Check sheet for the modelled part. Datum: model origin and axes. Units: mm. Face numbers are marked on the shaded views. Round coordinates to 2 decimals unless told otherwise and drop trailing zeros. Order: outer loops, then holes, each group sorted by start corner. A loop starts at its lowest first (then second) coordinate and runs counter-clockwise, first axis right, second up. Notation, with made-up numbers: (-29.5, -32) -> (28.5, -32) arc R17 ccw to (28.5, -11) -> close; hole circle Ø7 at (-10, 7.5). An arc over 180 degrees is marked (long way). Answer in a Markdown table with one row per item.
from build123d import *

# Parameters (mm, degrees)
PAD_DEPTH           = 3
PAD001_DEPTH        = 3.6
PAD002_DEPTH        = 5
HOLE001_D           = 3.3
HOLE001_DEPTH       = 25
HOLE001_CSINK_D     = 6
HOLE001_CSINK_ANGLE = 90
HOLE_D              = 3.3
HOLE_DEPTH          = 25
HOLE_CSINK_D        = 6
HOLE_CSINK_ANGLE    = 90


with BuildPart() as part:
    # Sketch → Pad (new body)
    with BuildSketch(Plane.XY):
        with BuildLine():
            Line((-31.5, 8.75), (-10.25, 8.75))
            ThreePointArc((-10.25, 8.75), (0, -1.5), (10.25, 8.75))
            Line((10.25, 8.75), (31.5, 8.75))
            Line((31.5, 8.75), (31.5, -8.75))
            Line((31.5, -8.75), (-31.5, -8.75))
            Line((-31.5, -8.75), (-31.5, 8.75))
        make_face()
    extrude(amount=PAD_DEPTH)

    # Sketch001 (on Face8 of Pad) → Pad001 (join)
    with BuildSketch(Plane.XY.offset(3)):
        Polygon((8.25, -5.539419), (16.5, 8.75), (31.5, 8.75), (31.5, -8.75), (-31.5, -8.75), (-31.5, 8.75), (-16.5, 8.75), (-8.25, -5.539419), align=None)
    extrude(amount=PAD001_DEPTH)

    # Sketch002 (on Face15 of Pad001) → Pad002 (join)
    with BuildSketch(Plane.XY.offset(6.6)):
        with BuildLine():
            Line((-31.5, 8.75), (-13.25, 8.75))
            ThreePointArc((-13.25, 8.75), (0, -4.5), (13.25, 8.75))
            Line((13.25, 8.75), (31.5, 8.75))
            Line((31.5, 8.75), (31.5, -8.75))
            Line((31.5, -8.75), (-31.5, -8.75))
            Line((-31.5, -8.75), (-31.5, 8.75))
        make_face()
    extrude(amount=PAD002_DEPTH)

    # Hole001
    with Locations(Plane.XY.offset(11.6)):
        with Locations((-22.54, -1.95), (22.54, -1.95)):
            CounterSinkHole(HOLE001_D / 2, HOLE001_CSINK_D / 2, depth=HOLE001_DEPTH, counter_sink_angle=HOLE001_CSINK_ANGLE)

    # Hole
    with Locations(Plane.XZ.offset(8.75)):
        with Locations((26.5, 4.5), (-26.5, 4.5)):
            CounterSinkHole(HOLE_D / 2, HOLE_CSINK_D / 2, depth=HOLE_DEPTH, counter_sink_angle=HOLE_CSINK_ANGLE)


solid = part.part
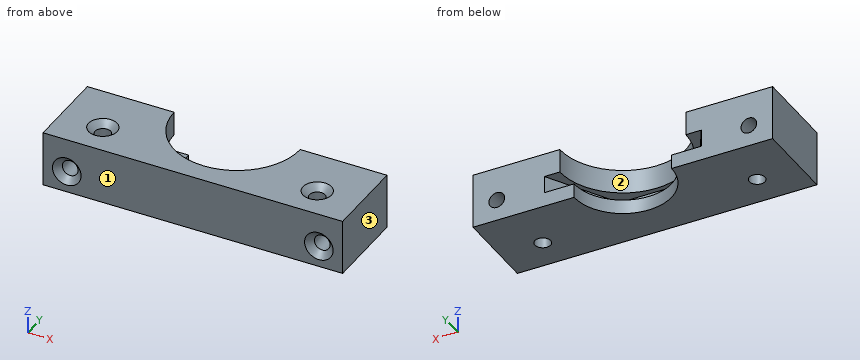
Item 1: Mould release check, pull along X, two halves, no side actions. Record for the marked faces 1, 2 and 3: pulls with the +X half, pulls with the -X half, needs draft (parallel to the pull), parting line crosses it, or undercut.
Result sheet:
| item | result |
|---|---|
| face 1 | needs draft |
| face 2 | undercut |
| face 3 | pulls with the +X half |
Item 2: Depth check by flat-ended pin: P1, Ø1.1, axis at x = 1.5, z = 5, coming from the +Y side; P2, Ø4, axis at x = 26.5, z = 4.5, coming from the -Y side; P3, Ø4, axis at x = 22.54, y = -1.95, coming from the +Z side; P4, Ø2, axis at x = -22.54, y = -1.95, coming from the +Z side. Enter the tip coordinate at first touch or a pass-through.
Result sheet:
| item | result |
|---|---|
| P1 | stops at y = -5.54 |
| P2 | stops at y = -7.75 |
| P3 | stops at z = 10.6 |
| P4 | passes through |
Item 3: Cross-section at B-B (x = -22.54). Record the boundary of the cut face in (y, z), and give its area (3 significant figures).
Result sheet:
| item | result |
|---|---|
| outline | (-8.75, 0) -> (-3.6, 0) -> (-3.6, 10.25) -> (-4.95, 11.6) -> (-8.75, 11.6) -> close; (-0.3, 0) -> (8.75, 0) -> (8.75, 11.6) -> (1.05, 11.6) -> (-0.3, 10.25) -> close |
| area | 163 mm^2 |
Item 4: Cross-section at D-D (y = 4.75). Record the boundary of the cut face in (x, z), and give its area (3 significant figures).
Result sheet:
| item | result |
|---|---|
| outline | (-31.5, 0) -> (-9.44, 0) -> (-9.44, 3) -> (-14.19, 3) -> (-14.19, 6.6) -> (-12.63, 6.6) -> (-12.63, 11.6) -> (-31.5, 11.6) -> close; (9.44, 0) -> (31.5, 0) -> (31.5, 11.6) -> (12.63, 11.6) -> (12.63, 6.6) -> (14.19, 6.6) -> (14.19, 3) -> (9.44, 3) -> close; hole circle Ø3.3 at (-26.5, 4.5); hole circle Ø3.3 at (26.5, 4.5) |
| area | 429 mm^2 |
Item 5: Scan lines: line 1 (X direction, y = -1.95, z = 2.5); line 2 (Y direction, x = -22.54, z = 7.75); line 3 (X direction, y = -1.5, z = 8.5). Record each from-to range of solid material in increasing order. Write a range as [from, to].
Result sheet:
| item | result |
|---|---|
| line 1 | x = [-31.5, -24.19], [-20.89, 20.89], [24.19, 31.5] |
| line 2 | y = [-8.75, -3.6], [-0.3, 8.75] |
| line 3 | x = [-31.5, -24.13], [-20.95, -8.4], [8.4, 20.95], [24.13, 31.5] |
Item 6: Cross-section at A-A (z = 4.5). Record the boundary of the cut face in (x, y).
Result sheet:
| item | result |
|---|---|
| outline | (-31.5, -8.75) -> (-29.5, -8.75) -> (-28.15, -7.4) -> (-28.15, 8.75) -> (-31.5, 8.75) -> close; (-24.85, -7.4) -> (-23.5, -8.75) -> (23.5, -8.75) -> (24.85, -7.4) -> (24.85, 8.75) -> (16.5, 8.75) -> (8.25, -5.54) -> (-8.25, -5.54) -> (-16.5, 8.75) -> (-24.85, 8.75) -> close; (28.15, -7.4) -> (29.5, -8.75) -> (31.5, -8.75) -> (31.5, 8.75) -> (28.15, 8.75) -> close; hole circle Ø3.3 at (-22.54, -1.95); hole circle Ø3.3 at (22.54, -1.95) |
Item 7: Cross-section at C-C (z = 8.75). Record the boundary of the cut face in (x, y), and give its area (3 significant figures).
Result sheet:
| item | result |
|---|---|
| outline | (-31.5, -8.75) -> (31.5, -8.75) -> (31.5, 8.75) -> (13.25, 8.75) arc R13.25 cw to (-13.25, 8.75) -> (-31.5, 8.75) -> close; hole circle Ø3.3 at (-22.54, -1.95); hole circle Ø3.3 at (22.54, -1.95) |
| area | 810 mm^2 |
